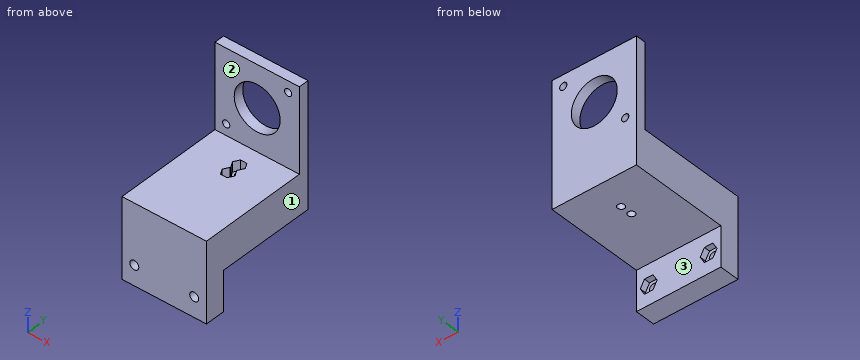
```python
from build123d import *

# Parameters (mm, degrees)
BOSS_EXTRUDE1_DEPTH = 42.25
SKETCH3_R           = 2.25
CUT_EXTRUDE1_DEPTH  = 78.46363663
SKETCH4_R           = 11.5
SKETCH4_R_2         = 1.8
CUT_EXTRUDE2_DEPTH  = 81.737940276
SKETCH5_R           = 1.75
CUT_EXTRUDE3_DEPTH  = 96.794650164
CUT_EXTRUDE4_DEPTH  = 5
CUT_EXTRUDE5_DEPTH  = 3


with BuildPart() as part:
    # Sketch1 → Boss-Extrude1 (new body)
    with BuildSketch(Plane(origin=(0, 0, 0), x_dir=(0, 0, -1), z_dir=(1, 0, 0))):
        Polygon((0, 0), (40, 0), (40, 10), (20, 10), (20, 59.3), (-42.25, 59.3), (-42.25, 54.3), (0, 54.3), align=None)
    extrude(amount=BOSS_EXTRUDE1_DEPTH)

    # Sketch3 → Cut-Extrude1 (cut, through all)
    with BuildSketch(Plane(origin=(0, 10, 0), x_dir=(1, 0, 0), z_dir=(0, 1, 0))):
        with Locations(Location((6.125, 30, 0), (0, 0, 270))):
            Circle(SKETCH3_R)
        with Locations(Location((36.125, 30, 0), (0, 0, 270))):
            Circle(SKETCH3_R)
    extrude(amount=-CUT_EXTRUDE1_DEPTH, mode=Mode.SUBTRACT)

    # Sketch4 → Cut-Extrude2 (cut, through all)
    with BuildSketch(Plane.XZ.offset(-54.3)):
        with Locations(Location((21.125, 21.125, 0), (0, 0, 270))):
            Circle(SKETCH4_R)
        with Locations(Location((5.625, 5.625, 0), (0, 0, 270))):
            Circle(SKETCH4_R_2)
        with Locations(Location((36.625, 36.625, 0), (0, 0, 270))):
            Circle(SKETCH4_R_2)
    extrude(amount=-CUT_EXTRUDE2_DEPTH, mode=Mode.SUBTRACT)

    # Sketch5 → Cut-Extrude3 (cut, through all)
    with BuildSketch(Plane(origin=(0, 0, -20), x_dir=(-1, 0, 0), z_dir=(0, 0, -1))):
        with Locations(Location((-21.125, 43.6, 0), (0, 0, 90))):
            Circle(SKETCH5_R)
        with Locations(Location((-21.125, 37.6, 0), (0, 0, 90))):
            Circle(SKETCH5_R)
    extrude(amount=-CUT_EXTRUDE3_DEPTH, mode=Mode.SUBTRACT)

    # Sketch6 → Cut-Extrude4 (cut)
    with BuildSketch(Plane.XY):
        Polygon((19.508419246, 40.8), (19.508419246, 40.4), (17.891838493, 37.6), (19.508419246, 34.8), (22.741580754, 34.8), (24.358161507, 37.6), (22.741580754, 40.4), (22.741580754, 40.8), (24.358161507, 43.6), (22.741580754, 46.4), (19.508419246, 46.4), (17.891838493, 43.6), align=None)
    extrude(amount=-CUT_EXTRUDE4_DEPTH, mode=Mode.SUBTRACT)

    # Sketch7 → Cut-Extrude5 (cut)
    with BuildSketch(Plane(origin=(0, 10, 0), x_dir=(1, 0, 0), z_dir=(0, 1, 0))):
        Polygon((10.339656965, 30), (8.232328483, 33.65), (4.017671517, 33.65), (1.910343035, 30), (4.017671517, 26.35), (8.232328483, 26.35), align=None)
        Polygon((40.339656965, 30), (38.232328483, 33.65), (34.017671517, 33.65), (31.910343035, 30), (34.017671517, 26.35), (38.232328483, 26.35), align=None)
    extrude(amount=-CUT_EXTRUDE5_DEPTH, mode=Mode.SUBTRACT)


solid = part.part
```
The listing builds one solid part. Answer for the finished solid, in the listing's coordinates (mm). Face numbers are marked on the shaded views. A direction names the side the tool comes from. Coordinates: 2 decimals unless noted, no trailing zeros. Write each loop counter-clockwise with the first axis right and the second up, starting at its lowest first coordinate (ties: lowest second). Pieces come first, ordered by that corner, then holes. Notation, with made-up numbers: (54, -6.5) - (77, -6.5) arc R21 cw to (77, 1.5) - close; hole circle Ø8 at (-33, 68.5). An arc over 180 degrees is marked (long way). One line per item, written item: value.
1) Find section C-C (z = -31). Give the vertices of the cut face in (x, y).
Geometry check:
outline: (0, 0) - (4.11, 0) - (4.11, 7) - (2.49, 7) - (2.49, 10) - (0, 10) - close; (8.14, 0) - (34.11, 0) - (34.11, 7) - (32.49, 7) - (32.49, 10) - (9.76, 10) - (9.76, 7) - (8.14, 7) - close; (38.14, 0) - (42.25, 0) - (42.25, 10) - (39.76, 10) - (39.76, 7) - (38.14, 7) - close
2) Find section D-D (y = 6). Give the vertices of the cut face in (x, z) (3 decimals).
Geometry check:
outline: (0, -40) - (42.25, -40) - (42.25, 0) - (0, 0) - close; hole circle Ø4.5 at (6.125, -30); hole circle Ø4.5 at (36.125, -30)
3) Each of these flat-tipped pins is pushed along its axis until it touches: pin 1 Ø6 at (x, y) = (6.5, 16) entering from +Z; pin 2 Ø22 at (x, z) = (26.5, -27) entering from +Y; pin 3 Ø6 at (x, z) = (34.5, -31) entering from +Y; pin 4 Ø3 at (x, z) = (30.5, 10) entering from -Y. Where does it stop, or does it pass through?
Geometry check:
pin 1: stops at z = 0
pin 2: stops at y = 59.3
pin 3: stops at y = 10
pin 4: stops at y = 54.3
4) Find section A-A (z = 27). Give the vertices of the cut face in (x, y).
Geometry check:
outline: (0, 54.3) - (11.24, 54.3) - (11.24, 59.3) - (0, 59.3) - close; (31.01, 54.3) - (42.25, 54.3) - (42.25, 59.3) - (31.01, 59.3) - close
5) A tool of negligible diameter and unlimited length cuts with its end or side. For the marked faces 1, 2 and 3, from which of +Z, -Z, +X, -X, +Y, -Y can it reach the whole face along a straight path? Write none if from no direction.
Geometry check:
face 1: +Z, -Z, +X, +Y, -Y
face 2: +Z, +X, -X, -Y
face 3: -Z, +X, -X, +Y
6) Consider line 1 along X through (y, z) = (5.75, -30) (3 decimals); line 2 along X through (y, z) = (37.6, -13) (3 decimals); line 3 along Z through (x, y) = (37, 14.5). Determine where each line is inside the solid, lowest interval first. Write a range as from..to.
Geometry check:
line 1: x = 0..3.875, 8.375..33.875, 38.375..42.25
line 2: x = 0..19.375, 22.875..42.25
line 3: z = -20..0
7) Find section B-B (x = 29). Give the vertices of the cut face in (y, z).
Geometry check:
outline: (0, -40) - (10, -40) - (10, -20) - (59.3, -20) - (59.3, 12.74) - (54.3, 12.74) - (54.3, 0) - (0, 0) - close; (54.3, 29.51) - (59.3, 29.51) - (59.3, 42.25) - (54.3, 42.25) - close
